from build123d import *

# Parameters (mm, degrees)
F0_W     = 54
F0_H     = 82
F0_R     = 2.5
F0_R_2   = 8
F1_DEPTH = 10
F2_SIZE  = 3
F3_W     = 30
F3_H     = 82
F4_DEPTH = 2
F5_R     = 0.5
F6_DEPTH = 27


with BuildPart() as f1:
    # F0 (on Top) → F1 (new body)
    with BuildSketch(Plane.XY):
        Rectangle(F0_W, F0_H)
        with Locations((-19, -33)):
            Circle(F0_R, mode=Mode.SUBTRACT)
        with Locations((0, -26)):
            Circle(F0_R_2, mode=Mode.SUBTRACT)
        with Locations((19, -33)):
            Circle(F0_R, mode=Mode.SUBTRACT)
        with Locations((-19, 0)):
            Circle(F0_R, mode=Mode.SUBTRACT)
        with Locations((-19, 33)):
            Circle(F0_R, mode=Mode.SUBTRACT)
        with Locations((19, 0)):
            Circle(F0_R, mode=Mode.SUBTRACT)
        with Locations((0, 26)):
            Circle(F0_R_2, mode=Mode.SUBTRACT)
        with Locations((19, 33)):
            Circle(F0_R, mode=Mode.SUBTRACT)
    extrude(amount=F1_DEPTH)

    # F2
    f2_edges = [f1.edges().sort_by_distance(p)[0] for p in [
        (27, -41, 5),
        (-27, -41, 5),
        (27, 41, 5),
        (-27, 41, 5),
    ]]
    chamfer(f2_edges, length=F2_SIZE)

    # F3 (on face) → F4 (cut)
    with BuildSketch(Plane.XY.offset(10)):
        Rectangle(F3_W, F3_H)
    extrude(amount=-F4_DEPTH, mode=Mode.SUBTRACT)

    # F5 (on face) → F6 (cut)
    with BuildSketch(Plane.YZ.offset(27)):
        with Locations((5, 7)):
            Circle(F5_R)
    extrude(amount=-F6_DEPTH, mode=Mode.SUBTRACT)


solid = f1.part
Verification items for the finished model (mm, model axes). A direction names the side the tool comes from. Coordinates: 2 decimals unless noted, no trailing zeros. Loops run counter-clockwise (first coordinate to the right, second up) from the corner with the lowest first, then second, coordinate; pieces in that order, holes last. Notation, with made-up numbers: (87, 6) -> (94, 6) arc R30 cw to (94, 42) -> close; hole circle Ø1 at (-10.5, 65.5). An arc over 180 degrees is marked (long way). Answer as a JSON object with one key per item and string values. Group by question number.
Item 1: Sectioned sample at C-C on z = 4. State how many separate pieces and enclosed holes the cut face has, plus the area to 3 significant figures.
Item 2: Sectioned sample at A-A on y = -26. Record the boundary of the cut face in (x, z), plus the area to 3 significant figures.
Item 3: Tool access check on faces 1 (the cylindrical face through (-20.84, -31.31, 4.93)), 2 (the flat face through (0, 1, 8)). Record the directions out of +Z, -Z, +X, -X, +Y, -Y that give a thin tool (end or side, any length) a straight path to the whole face; none if there is none.
Item 4: Sectioned sample at D-D on y = 13. Record the boundary of the cut face in (x, z).
Item 5: Sectioned sample at B-B on x = 3. Record the boundary of the cut face in (y, z), plus the area to 3 significant figures.
Item 6: Mould release check, pull along Y, two halves, no side actions. Record for faces 3 (the flat face through (22, 1, 10)), 4 (the cylindrical face through (16.5, 0.1, 4.9)), 5 (the cylindrical face through (-21.5, 0.1, 4.9)), 6 (the flat face through (-25, 40, 5)): +Y half, -Y half, draft (parallel to the pull), parting line (faces both ways), or undercut.
Item 7: Scan lines: probe 1 along Y at (x, z) = (-19, 3); probe 2 along Z at (x, y) = (21.75, 5); probe 3 along Z at (x, y) = (11.5, 5). Record each from-to range of solid material in increasing order.
Item 8: Depth check by flat-ended pin: pin 1 (2 mm diameter, centred on x = 9.5, y = 21.5, fed in from +Z); pin 2 (0.8 mm diameter, centred on y = 5, z = 7, fed in from +X). Enter the tip coordinate at first touch or a pass-through.
Evaluation:
{
 "1": {"separate pieces": "1", "enclosed holes": "8", "area": "3,890 mm²"},
 "2": {"outline": "(-27, 0) -> (-8, 0) -> (-8, 8) -> (-15, 8) -> (-15, 10) -> (-27, 10) -> close; (8, 0) -> (27, 0) -> (27, 10) -> (15, 10) -> (15, 8) -> (8, 8) -> close", "area": "352 mm²"},
 "3": {"face 1": "+Z, -Z", "face 2": "+Z, +Y, -Y"},
 "4": {"outline": "(-27, 0) -> (27, 0) -> (27, 10) -> (15, 10) -> (15, 8) -> (-15, 8) -> (-15, 10) -> (-27, 10) -> close"},
 "5": {"outline": "(-41, 0) -> (-33.42, 0) -> (-33.42, 8) -> (-41, 8) -> close; (-18.58, 0) -> (18.58, 0) -> (18.58, 8) -> (-18.58, 8) -> close; (33.42, 0) -> (41, 0) -> (41, 8) -> (33.42, 8) -> close; hole circle Ø1 at (5, 7)", "area": "418 mm²"},
 "6": {"face 3": "draft", "face 4": "undercut", "face 5": "undercut", "face 6": "+Y half"},
 "7": {"probe 1": "y = -41 to -35.5, -30.5 to -2.5, 2.5 to 30.5, 35.5 to 41", "probe 2": "z = 0 to 6.5, 7.5 to 10", "probe 3": "z = 0 to 6.5, 7.5 to 8"},
 "8": {"pin 1": "stops at z = 8", "pin 2": "stops at x = 0"}
}
